The drawing under review shows one solid part. Ordinate dimensions are in mm from its lowest x, y, z. A direction names the side the tool comes from. Coordinates: 2 decimals unless noted, no trailing zeros. Write each loop counter-clockwise with the first axis right and the second up, starting at its lowest first coordinate (ties: lowest second). Pieces come first, ordered by that corner, then holes. Notation, with made-up numbers: (46, 67.25) - (66, 67.25) arc R26 ccw to (66, 98.25) - close; hole circle Ø1 at (3.25, -10). An arc over 180 degrees is marked (long way). Put each result on its own line as item: value. Start each with the question number.
Item 1: For pin 1 (10 mm diameter, centred on x = 41.5, y = 24.5, fed in from +Z), flat-tipped, find the tip position at first contact; note if it passes through.
Item 2: To check wall thickness, follow L1, parallel to X at y = 115.5, z = 46.5 (1 decimal); L2, parallel to Y at x = 15.5, z = 15.5 (1 decimal); L3, parallel to Y at x = 63, z = 40. State the ranges of each line that lie inside material, in increasing order. Write a range as [from, to].
Item 3: Consider section A-A on x = 60. Give the boundary of the cut face in (y, z), then the cut area to 3 significant figures.
Item 4: Consider section D-D on y = 28.5. Give the boundary of the cut face in (x, z).
Item 5: Consider section C-C on x = 43. Give the boundary of the cut face in (y, z).
Item 6: Machinability: for the marked faces 1 and 2, which of the approach directions +Z, -Z, +X, -X, +Y, -Y give a long, thin tool a straight path to every point of the face, cutting with its end or side? Answer none if there is none.
Item 7: Consider section B-B on z = 20.5. State how many separate pieces and enclosed holes the cut face has, then the cut area to 3 significant figures.
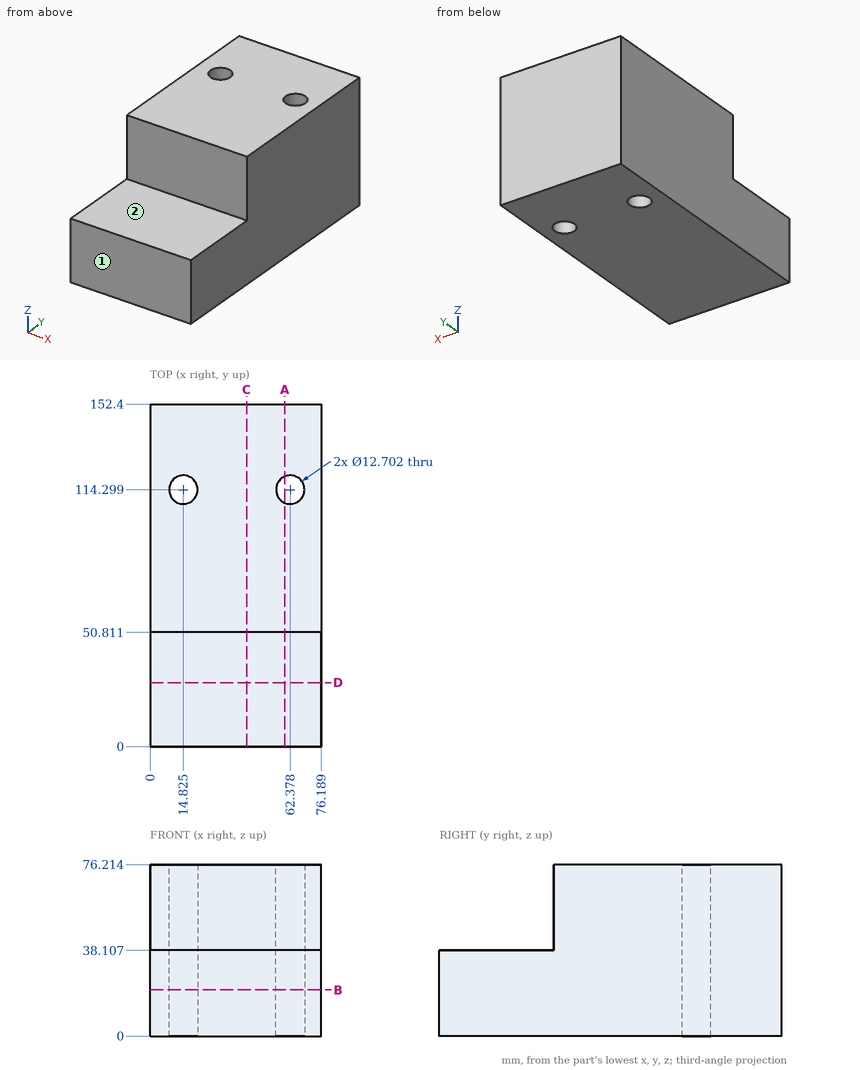
Report:
1. pin 1: z = 38.11
2. L1: [0, 8.6], [21.1, 56.1], [68.6, 76.2]
2. L2: [0, 108], [120.6, 152.4]
2. L3: [50.81, 107.98], [120.62, 152.4]
3. outline: (0, 0) - (108.41, 0) - (108.41, 76.21) - (50.81, 76.21) - (50.81, 38.11) - (0, 38.11) - close; (120.19, 0) - (152.4, 0) - (152.4, 76.21) - (120.19, 76.21) - close
3. area: 8,780 mm²
4. outline: (0, 0) - (76.19, 0) - (76.19, 38.11) - (0, 38.11) - close
5. outline: (0, 0) - (152.4, 0) - (152.4, 76.21) - (50.81, 76.21) - (50.81, 38.11) - (0, 38.11) - close
6. face 1: +Z, -Z, +X, -X, -Y
6. face 2: +Z, +X, -X, -Y
7. separate pieces: 1
7. enclosed holes: 2
7. area: 11,400 mm²
